```python
from build123d import *

# Parameters (mm, degrees)
F0_R     = 41
F0_R_2   = 26
F1_DEPTH = 177.5
F2_R     = 30
F2_R_2   = 26
F3_DEPTH = 220


with BuildPart() as f1:
    # F0 (on Top) → F1 (new body)
    with BuildSketch(Plane.XY):
        Circle(F0_R)
        Circle(F0_R_2, mode=Mode.SUBTRACT)
    extrude(amount=F1_DEPTH)

    # F2 (on Top) → F3 (join)
    with BuildSketch(Plane.XY):
        Circle(F2_R)
        Circle(F2_R_2, mode=Mode.SUBTRACT)
    extrude(amount=-F3_DEPTH)


solid = f1.part
```
CAD build for the part. Positions are in the model's coordinates, mm. A direction names the side the tool comes from. Round coordinates to 2 decimals unless told otherwise and drop trailing zeros. Loops run counter-clockwise (first coordinate to the right, second up) from the corner with the lowest first, then second, coordinate; pieces in that order, holes last. Notation, with made-up numbers: (85, 11.5) - (128, 11.5) arc R13 ccw to (128, 31.5) - close; hole circle Ø1 at (8, 65.25). An arc over 180 degrees is marked (long way). Return JSON: item names as keys, results as strings. Group by question number.
Q1. Band-saw the part on D-D on z = 95.5. Give the cut face in (x, y).
Q2. Band-saw the part on C-C on z = -151.5. Give the cut face in (x, y).
Q3. Tool access for faces 1 (the face through (2.8, -30.2, 0)), 2 (the face through (-9, -40, 88)): list every direction of +Z, -Z, +X, -X, +Y, -Y with a clear straight run to the whole face (end or side of a thin tool).
Q4. Band-saw the part on A-A on y = 0. Give the cut face in (x, z), plus the area to 4 significant figures.
Q5. Drill centre lines: line 1 along Y through (x, z) = (0, 66.5); line 2 along Z through (x, y) = (4, 34); line 3 along Y through (x, z) = (22, -74). Where is each one in solid material? Low to high. Write a range as [from, to].
Q6. Flat gauge pins, fed straight in: pin 1 Ø10 at (x, y) = (-19.5, -16) entering from -Z; pin 2 Ø6 at (x, z) = (5.5, 19) entering from +Y; pin 3 Ø12 at (x, z) = (-11, 31.5) entering from -Y; pin 4 Ø8 at (y, z) = (10, -139.5) entering from +X. Where does each tip first touch, or does it go through?
Solutions:
{
 "1": {"outline": "circle Ø82 at (0, 0); hole circle Ø52 at (0, 0)"},
 "2": {"outline": "circle Ø60 at (0, 0); hole circle Ø52 at (0, 0)"},
 "3": {"face 1": "-Z", "face 2": "+Z, -Z"},
 "4": {"outline": "(-41, 0) - (-30, 0) - (-30, -220) - (-26, -220) - (-26, 177.5) - (-41, 177.5) - close; (26, -220) - (30, -220) - (30, 0) - (41, 0) - (41, 177.5) - (26, 177.5) - close", "area": "7,085 mm^2"},
 "5": {"line 1": "y = [-41, -26], [26, 41]", "line 2": "z = [0, 177.5]", "line 3": "y = [-20.4, -13.86], [13.86, 20.4]"},
 "6": {"pin 1": "stops at z = -220", "pin 2": "stops at y = 40.92", "pin 3": "stops at y = -40.69", "pin 4": "stops at x = 29.39"}
}
